Can you work these out from the model? Positions are in its coordinate system, mm. Round coordinates to 2 decimals unless told otherwise and drop trailing zeros. Write each loop counter-clockwise with the first axis right and the second up, starting at its lowest first coordinate (ties: lowest second). Pieces come first, ordered by that corner, then holes. Notation, with made-up numbers: M -21,69.5 L 14,69.5 A25 ccw 14,106.5 Z; hole C 72,71 d8. An arc over 180 degrees is marked long. Answer in a Markdown table with one row per item. Add a question column.
(1) Suppose I cut it at C-C, the plane y = 1.75. Write out the boundary of the cut face in (x, z), then the cut area to 3 significant figures.
(2) If I drill on probe 1 along X at (y, z) = (-0.6, 0); probe 2 along X at (y, z) = (2.85, 0); probe 3 along Z at (x, y) = (-2, 1.25), over which ranges is the centre line in solid material (lowest first)?
(3) Suppose I cut it at D-D, the plane x = -24.5. Write out the boundary of the cut face in (y, z), then the cut area to 3 significant figures.
(4) Suppose I cut it at A-A, the plane x = 0. Write out the boundary of the cut face in (y, z), then the cut area to 3 significant figures.
(5) I'm going to push flat-ended pins straight in: pin 1 (4 mm diameter, centred on x = 20.5, y = 2.5, fed in from +Z); pin 2 (9 mm diameter, centred on x = 0, z = 0, fed in from -Y); pin 3 (0.8 mm diameter, centred on y = 2, z = -5.5, fed in from +X); pin 4 (1 mm diameter, centred on x = 29.5, y = 2.5, fed in from +Z). Where does each tip first touch, or does it pass through?
(6) Suppose I cut it at B-B, the plane z = -1. Write out the boundary of the cut face in (x, y), then the cut area to 3 significant figures.
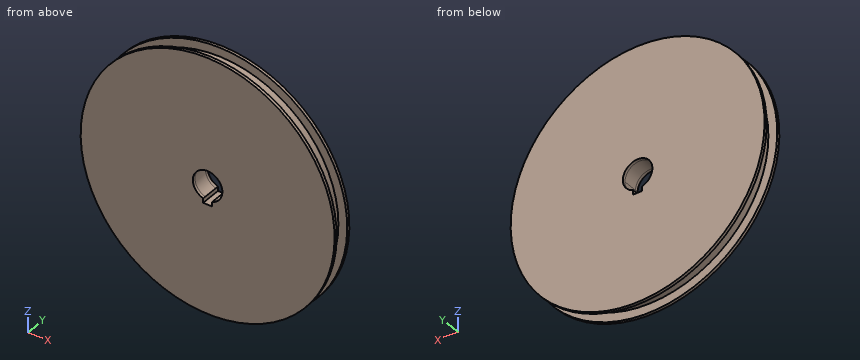
from build123d import *

# Parameters (mm, degrees)
SKETCH1_R           = 40
BOSS_EXTRUDE1_DEPTH = 5
BOSS_EXTRUDE2_START = -1
SKETCH1_3_R         = 43
BOSS_EXTRUDE2_DEPTH = 1
BOSS_EXTRUDE3_START = 5
SKETCH1_4_R         = 43
BOSS_EXTRUDE3_DEPTH = 1


with BuildPart() as part:
    # Sketch1 → Boss-Extrude1 (new body)
    with BuildSketch(Plane(origin=(0, 0, 0), x_dir=(1, 0, 0), z_dir=(0, 1, 0))):
        with Locations(Location((0, 0, 0), (0, 0, 270))):
            Circle(SKETCH1_R)
        with BuildLine():
            ThreePointArc((5, 0), (-2.958039892, -4.031128874), (-1.5, 4.769696007))
            Line((-1.5, 4.769696007), (-1.5, 6.269696007))
            Line((-1.5, 6.269696007), (1.5, 6.269696007))
            Line((1.5, 6.269696007), (1.5, 4.769696007))
            ThreePointArc((1.5, 4.769696007), (4.031128874, 2.958039892), (5, 0))
        make_face(mode=Mode.SUBTRACT)
    extrude(amount=BOSS_EXTRUDE1_DEPTH)

    # Sketch1<3> → Boss-Extrude2 (add)
    with BuildSketch(Plane(origin=(0, 0, 0), x_dir=(1, 0, 0), z_dir=(0, 1, 0)).offset(BOSS_EXTRUDE2_START)):
        with Locations(Location((0, 0, 0), (0, 0, 270))):
            Circle(SKETCH1_3_R)
        with BuildLine():
            Line((-1.5, 4.769696007), (-1.5, 6.269696007))
            Line((-1.5, 6.269696007), (1.5, 6.269696007))
            Line((1.5, 6.269696007), (1.5, 4.769696007))
            ThreePointArc((1.5, 4.769696007), (0, -5), (-1.5, 4.769696007))
        make_face(mode=Mode.SUBTRACT)
    extrude(amount=BOSS_EXTRUDE2_DEPTH)

    # Sketch1<4> → Boss-Extrude3 (add)
    with BuildSketch(Plane(origin=(0, 0, 0), x_dir=(1, 0, 0), z_dir=(0, 1, 0)).offset(BOSS_EXTRUDE3_START)):
        with Locations(Location((0, 0, 0), (0, 0, 270))):
            Circle(SKETCH1_4_R)
        with BuildLine():
            Line((-1.5, 4.769696007), (-1.5, 6.269696007))
            Line((-1.5, 6.269696007), (1.5, 6.269696007))
            Line((1.5, 6.269696007), (1.5, 4.769696007))
            ThreePointArc((1.5, 4.769696007), (0, -5), (-1.5, 4.769696007))
        make_face(mode=Mode.SUBTRACT)
    extrude(amount=BOSS_EXTRUDE3_DEPTH)


solid = part.part
Calculated:
| question | item | result |
|---|---|---|
| 1 | outline | C 0,0 d80; hole M -1.5,-6.27 L 1.5,-6.27 L 1.5,-4.77 A5 ccw long -1.5,-4.77 Z |
| 1 | area | 4,940 mm² |
| 2 | probe 1 | -43 to -5, 5 to 43 |
| 2 | probe 2 | -40 to -5, 5 to 40 |
| 2 | probe 3 | -39.95 to -4.58, 4.58 to 39.95 |
| 3 | outline | M -1,-35.34 L 0,-35.34 L 0,-31.62 L 5,-31.62 L 5,-35.34 L 6,-35.34 L 6,35.34 L 5,35.34 L 5,31.62 L 0,31.62 L 0,35.34 L -1,35.34 Z |
| 3 | area | 458 mm² |
| 4 | outline | M -1,-43 L 0,-43 L 0,-40 L 5,-40 L 5,-43 L 6,-43 L 6,-6.27 L -1,-6.27 Z; M -1,5 L 6,5 L 6,43 L 5,43 L 5,40 L 0,40 L 0,43 L -1,43 Z |
| 4 | area | 493 mm² |
| 5 | pin 1 | z = 35.46 |
| 5 | pin 2 | through |
| 5 | pin 3 | x = 39.67 |
| 5 | pin 4 | z = 27.55 |
| 6 | outline | M -42.99,-1 L -4.9,-1 L -4.9,6 L -42.99,6 L -42.99,5 L -39.99,5 L -39.99,0 L -42.99,0 Z; M 4.9,-1 L 42.99,-1 L 42.99,0 L 39.99,0 L 39.99,5 L 42.99,5 L 42.99,6 L 4.9,6 Z |
| 6 | area | 503 mm² |
